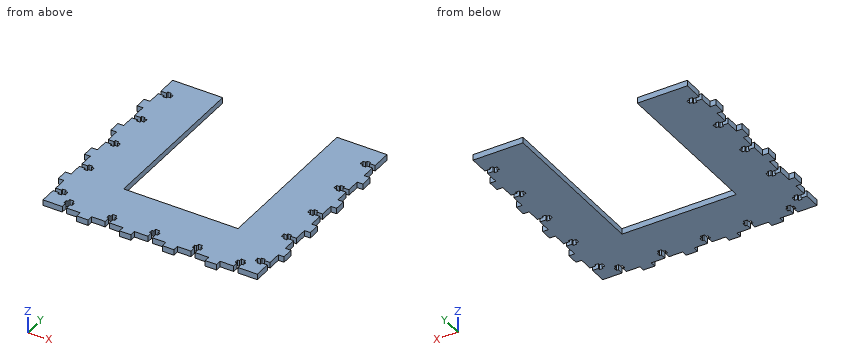
from build123d import *

# Parameters (mm, degrees)
EXTRUDE_1_DEPTH     = 4
SKETCH_4_W          = 80
SKETCH_4_H          = 113
CUT_EXTRUDE_1_DEPTH = 4


with BuildPart() as part:
    # 草图1 → 凸台-拉伸1 (new body)
    with BuildSketch(Plane.XY):
        Polygon((145, 56.5), (149, 56.5), (149, 55.15), (151.6, 55.15), (151.6, 56.5), (153.6, 56.5), (153.6, 59.5), (151.6, 59.5), (151.6, 60.85), (149, 60.85), (149, 59.5), (145, 59.5), (145, 69), (141, 69), (141, 77), (145, 77), (145, 86.5), (149, 86.5), (149, 85.15), (151.6, 85.15), (151.6, 86.5), (153.6, 86.5), (153.6, 89.5), (151.6, 89.5), (151.6, 90.85), (149, 90.85), (149, 89.5), (145, 89.5), (145, 99), (141, 99), (141, 107), (145, 107), (145, 116.5), (149, 116.5), (149, 115.15), (151.6, 115.15), (151.6, 116.5), (153.6, 116.5), (153.6, 119.5), (151.6, 119.5), (151.6, 120.85), (149, 120.85), (149, 119.5), (145, 119.5), (145, 133), (295, 133), (295, 119.5), (291, 119.5), (291, 120.85), (288.4, 120.85), (288.4, 119.5), (286.4, 119.5), (286.4, 116.5), (288.4, 116.5), (288.4, 115.15), (291, 115.15), (291, 116.5), (295, 116.5), (295, 107), (299, 107), (299, 99), (295, 99), (295, 89.5), (291, 89.5), (291, 90.85), (288.4, 90.85), (288.4, 89.5), (286.4, 89.5), (286.4, 86.5), (288.4, 86.5), (288.4, 85.15), (291, 85.15), (291, 86.5), (295, 86.5), (295, 77), (299, 77), (299, 69), (295, 69), (295, 59.5), (291, 59.5), (291, 60.85), (288.4, 60.85), (288.4, 59.5), (286.4, 59.5), (286.4, 56.5), (288.4, 56.5), (288.4, 55.15), (291, 55.15), (291, 56.5), (295, 56.5), (295, 47), (299, 47), (299, 39), (295, 39), (295, 29.5), (291, 29.5), (291, 30.85), (288.4, 30.85), (288.4, 29.5), (286.4, 29.5), (286.4, 26.5), (288.4, 26.5), (288.4, 25.15), (291, 25.15), (291, 26.5), (295, 26.5), (295, 17), (299, 17), (299, 9), (295, 9), (295, -0.5), (291, -0.5), (291, 0.85), (288.4, 0.85), (288.4, -0.5), (286.4, -0.5), (286.4, -3.5), (288.4, -3.5), (288.4, -4.85), (291, -4.85), (291, -3.5), (295, -3.5), (295, -15), (281.5, -15), (281.5, -11), (282.85, -11), (282.85, -8.4), (281.5, -8.4), (281.5, -6.4), (278.5, -6.4), (278.5, -8.4), (277.15, -8.4), (277.15, -11), (278.5, -11), (278.5, -15), (269, -15), (269, -19), (261, -19), (261, -15), (251.5, -15), (251.5, -11), (252.85, -11), (252.85, -8.4), (251.5, -8.4), (251.5, -6.4), (248.5, -6.4), (248.5, -8.4), (247.15, -8.4), (247.15, -11), (248.5, -11), (248.5, -15), (239, -15), (239, -19), (231, -19), (231, -15), (221.5, -15), (221.5, -11), (222.85, -11), (222.85, -8.4), (221.5, -8.4), (221.5, -6.4), (218.5, -6.4), (218.5, -8.4), (217.15, -8.4), (217.15, -11), (218.5, -11), (218.5, -15), (209, -15), (209, -19), (201, -19), (201, -15), (191.5, -15), (191.5, -11), (192.85, -11), (192.85, -8.4), (191.5, -8.4), (191.5, -6.4), (188.5, -6.4), (188.5, -8.4), (187.15, -8.4), (187.15, -11), (188.5, -11), (188.5, -15), (179, -15), (179, -19), (171, -19), (171, -15), (161.5, -15), (161.5, -11), (162.85, -11), (162.85, -8.4), (161.5, -8.4), (161.5, -6.4), (158.5, -6.4), (158.5, -8.4), (157.15, -8.4), (157.15, -11), (158.5, -11), (158.5, -15), (145, -15), (145, -3.5), (149, -3.5), (149, -4.85), (151.6, -4.85), (151.6, -3.5), (153.6, -3.5), (153.6, -0.5), (151.6, -0.5), (151.6, 0.85), (149, 0.85), (149, -0.5), (145, -0.5), (145, 9), (141, 9), (141, 17), (145, 17), (145, 26.5), (149, 26.5), (149, 25.15), (151.6, 25.15), (151.6, 26.5), (153.6, 26.5), (153.6, 29.5), (151.6, 29.5), (151.6, 30.85), (149, 30.85), (149, 29.5), (145, 29.5), (145, 39), (141, 39), (141, 47), (145, 47), align=None)
    extrude(amount=EXTRUDE_1_DEPTH)

    # 草图4 → 切除-拉伸1 (cut)
    with BuildSketch(Plane(origin=(0, 0, 0), x_dir=(-1, 0, 0), z_dir=(0, 0, -1))):
        with Locations((-220, 76.5)):
            Rectangle(SKETCH_4_W, SKETCH_4_H)
    extrude(amount=-CUT_EXTRUDE_1_DEPTH, mode=Mode.SUBTRACT)


solid = part.part
Could you check a few things on this model? Use its own coordinates, in mm. Give positions to 0.01 mm unless a question says otherwise; leave off trailing zeros. Order: outer loops, then holes, each group sorted by start corner. A loop starts at its lowest first (then second) coordinate and runs counter-clockwise, first axis right, second up. Notation, with made-up numbers: (73, -7) -> (94, -7) arc R25 cw to (94, 31) -> close; hole circle Ø7 at (-9, 35). An arc over 180 degrees is marked (long way). Return JSON: item names as keys, results as strings.
1. For pin 1 Ø2 at (x, z) = (142.5, 3) entering from +Y; pin 2 Ø2 at (x, z) = (293.5, 1.5) entering from -Y; pin 3 Ø2 at (y, z) = (66, 3) entering from -X; pin 4 Ø4 at (x, y) = (163.5, 58) entering from -Z, each with a flat end and sliding along its axis, tell me the tip position at first contact or that it passes through.
Answer list:
{"pin 1": "stops at y = 107", "pin 2": "stops at y = -15", "pin 3": "stops at x = 145", "pin 4": "stops at z = 0"}
2. Imagine slicing it at B-B on x = 227.5. List the corners of the cut face in (y, z) for me, then the cut area to 3 significant figures.
Answer list:
{"outline": "(-15, 0) -> (20, 0) -> (20, 4) -> (-15, 4) -> close", "area": "140 mm2"}
3. I need wall thicknesses on line 1 (X direction, y = -9, z = 2.2); line 2 (X direction, y = 90, z = 3.85); line 3 (X direction, y = 49.5, z = 2). Which ranges of each line are inside material? Lowest first, please. Write a range as from..to.
Answer list:
{"line 1": "x = 145..157.15, 162.85..187.15, 192.85..217.15, 222.85..247.15, 252.85..277.15, 282.85..295", "line 2": "x = 145..149, 151.6..180, 260..288.4, 291..295", "line 3": "x = 145..180, 260..295"}
4. Imagine slicing it at A-A on y = 81. List the corners of the cut face in (x, z) for me.
Answer list:
{"outline": "(145, 0) -> (180, 0) -> (180, 4) -> (145, 4) -> close; (260, 0) -> (295, 0) -> (295, 4) -> (260, 4) -> close"}
